Design review of the part built by this model. Coordinates are the model's own, in mm. A direction names the side the tool comes from. Give positions to 0.01 mm unless a question says otherwise; leave off trailing zeros. Loops run counter-clockwise (first coordinate to the right, second up) from the corner with the lowest first, then second, coordinate; pieces in that order, holes last. Notation, with made-up numbers: (11, 58.25) - (67, 58.25) arc R33 ccw to (67, 97.25) - close; hole circle Ø10 at (23, -5.5). An arc over 180 degrees is marked (long way). Write each question's results on one line, items separated by ' | '.
```python
from build123d import *

# Parameters (mm, degrees)
CROQUIS1_R              = 1.5
SALIENTE_EXTRUIR1_DEPTH = 3
CROQUIS2_R              = 8.5
CORTAR_EXTRUIR1_DEPTH   = 1


with BuildPart() as part:
    # Croquis1 → Saliente-Extruir1 (new body)
    with BuildSketch(Plane.XY):
        with BuildLine():
            Line((-113.991811363, 10.970788205), (-113.991811363, 34.958108792))
            Line((-113.991811363, 34.958108792), (-123.991811363, 34.958108792))
            Line((-123.991811363, 34.958108792), (-123.991811363, 82.236637471))
            Line((-123.991811363, 82.236637471), (-63.991811363, 82.236637471))
            Line((-63.991811363, 82.236637471), (-63.991811363, 37.236637471))
            Line((-63.991811363, 37.236637471), (-73.991811363, 37.236637471))
            Line((-73.991811363, 37.236637471), (-73.991811363, 10.970788205))
            ThreePointArc((-73.991811363, 10.970788205), (-93.991811363, -9.029211795), (-113.991811363, 10.970788205))
        make_face()
        with Locations((-93.991811363, 10.970788205)):
            Circle(CROQUIS1_R, mode=Mode.SUBTRACT)
    extrude(amount=SALIENTE_EXTRUIR1_DEPTH)

    # Croquis2 → Cortar-Extruir1 (cut)
    with BuildSketch(Plane.XY.offset(3)):
        with Locations((-93.991811363, 10.970788205)):
            Circle(CROQUIS2_R)
    extrude(amount=-CORTAR_EXTRUIR1_DEPTH, mode=Mode.SUBTRACT)


solid = part.part
```
Item 1: We need section D-D on y = 21. Give the boundary of the cut face in (x, z), then the cut area to 3 significant figures.
Output values:
outline: (-113.99, 0) - (-73.99, 0) - (-73.99, 3) - (-113.99, 3) - close | area: 120 mm²
Item 2: Draft analysis for pull direction X (two halves, no side actions). For faces 6 (the face through (-113.992, 23, 1)), 7 (the face through (-85.884, 13.524, 2.507)), 8 (the face through (-69, 37.237, 1)), 9 (the face through (-95.49, 11.04, 0.99)), state which applies: +X half, -X half, draft (parallel to the pull), parting line (faces both ways), or undercut.
Output values:
face 6: -X half | face 7: undercut | face 8: draft | face 9: undercut
Item 3: Clearance check with flat-ended pins moving along their axes: P1, Ø4, axis at x = -93.99, y = 10.97, coming from the +Z side; P2, Ø0.9, axis at x = -67, z = 2, coming from the -Y side; P3, Ø1.5, axis at y = 24.5, z = 1, coming from the -X side; P4, Ø22, axis at x = -93.99, y = 10.97, coming from the -Z side. State where each tip first meets the part, or that it passes through.
Output values:
P1: stops at z = 2 | P2: stops at y = 37.24 | P3: stops at x = -113.99 | P4: stops at z = 0
Item 4: We need section A-A on z = 2.45. Give the boundary of the cut face in (x, y).
Output values:
outline: (-123.99, 34.96) - (-113.99, 34.96) - (-113.99, 10.97) arc R20 ccw to (-73.99, 10.97) - (-73.99, 37.24) - (-63.99, 37.24) - (-63.99, 82.24) - (-123.99, 82.24) - close; hole circle Ø17 at (-93.99, 10.97)
Item 5: Wall thickness on probe 1 along Y at (x, z) = (-98, 2.3); probe 2 along Y at (x, z) = (-70, 0.5); probe 3 along Y at (x, z) = (-93.5, 0.25): over which ranges is each line inside the solid? List them lowest first.
Output values:
probe 1: y = -8.62 to 3.48, 18.47 to 82.24 | probe 2: y = 37.24 to 82.24 | probe 3: y = -9.02 to 9.55, 12.39 to 82.24
Item 6: We need section B-B on y = 6.5. Give the boundary of the cut face in (x, z).
Output values:
outline: (-113.49, 0) - (-74.5, 0) - (-74.5, 3) - (-86.76, 3) - (-86.76, 2) - (-101.22, 2) - (-101.22, 3) - (-113.49, 3) - close
Item 7: We need section C-C on x = -89.5. Give the boundary of the cut face in (y, z), then the cut area to 3 significant figures.
Output values:
outline: (-8.52, 0) - (82.24, 0) - (82.24, 3) - (18.19, 3) - (18.19, 2) - (3.75, 2) - (3.75, 3) - (-8.52, 3) - close | area: 258 mm²
Item 8: Tool access review of faces 1 (the face through (-94, 9, 2)), 2 (the face through (-94, 47, 3)), 3 (the face through (-73.992, 24, 1)), 4 (the face through (-119, 34.958, 1)), 5 (the face through (-94, 82.237, 1)): name each direction out of +Z, -Z, +X, -X, +Y, -Y from which nothing blocks a thin tool from reaching the whole face with its end or side.
Output values:
face 1: +Z | face 2: +Z, +X, -X, +Y, -Y | face 3: +Z, -Z, +X, -Y | face 4: +Z, -Z, -X, -Y | face 5: +Z, -Z, +X, -X, +Y
